Source: CAD feature listing. Evaluate the final solid. Frame: model axes, mm. A direction names the side the tool comes from. Give positions to 0.01 mm unless a question says otherwise; leave off trailing zeros. Loops run counter-clockwise (first coordinate to the right, second up) from the corner with the lowest first, then second, coordinate; pieces in that order, holes last. Notation, with made-up numbers: (46.25, 55.5) - (93.25, 55.5) arc R5 cw to (93.25, 62.5) - close; hole circle Ø7 at (-6, 11). An arc over 180 degrees is marked (long way). Write each question's results on one line, items separated by ' | '. Start each with the question number.
(1) Material intervals for line 1 along Z through (x, y) = (-10.6, 5); line 2 along X through (y, z) = (7, 19.25); line 3 along Y through (x, z) = (10.85, 15), sorted ascending. Write a range as [from, to].
(2) Contact query for flat-ended pins moving along their axis: pin 1 (3.5 mm diameter, centred on x = 0, z = 27, fed in from -Y); pin 2 (3 mm diameter, centred on x = 0.5, z = 26.5, fed in from +Y); pin 3 (1.5 mm diameter, centred on y = 0, z = 27, fed in from +X); pin 4 (1.6 mm diameter, centred on x = -9.5, z = 15, fed in from +Y). Output: stop coordinate, or through.
(3) Pull-direction query (X, two-part tool) for faces 6 (the cylindrical face through (3.4, 0.52, 30.43)), 7 (the cylindrical face through (10.62, 9.289, 6.025)), 8 (the flat face through (0, 1, 22)); classes: pulls with the +X half, pulls with the -X half, needs draft (parallel to the pull), parting line crosses it, or undercut.
(4) Cut plane C-C on x = 1. Return the cut outline in (y, z).
(5) Cut plane D-D on y = 9.25. Return the cut outline in (x, z), then the cut area to 3 significant figures.
(6) Cut plane B-B on y = 5.75. Return the cut outline in (x, z), then the cut area to 3 significant figures.
(7) Reachability of faces 1 (the flat face through (9, 0, 13)), 2 (the flat face through (4, 0, 27)), 3 (the flat face through (-1.396, 1.014, 24.63)), 4 (the flat face through (-1, -1, 23)), 5 (the flat face through (-0.2, 2.4, 23)) from +Z, -Z, +X, -X, +Y, -Y: full face, straight path, thin tool, end or side. Return the list, or none.
(8) Cut plane A-A on z = 14. Return the cut outline in (x, y).
Autodesk Inventor part; units mm, degrees
ref_plane "YZ Plane" through (0, 0, 0) normal (1, 0, 0) x (0, 1, 0)
ref_plane "XZ Plane" through (0, 0, 0) normal (0, 1, 0) x (-1, 0, 0)
ref_plane "XY Plane" through (0, 0, 0) normal (0, 0, 1) x (1, 0, 0)
sketch "Sketch1" plane through (0, 0, 0) normal (0, 1, 0) x (-1, 0, 0)
  line L0 (10.25, 22) -> (-10.25, 22)
  line L1 (-10.25, 22) -> (-10.25, -22)
  line L2 (-10.25, -22) -> (10.25, -22)
  line L3 (10.25, -22) -> (10.25, 22)
  line L4 (10.25, 22) -> (-10.25, -22) construction
  line L5 (-10.25, 22) -> (10.25, -22) construction
  line L6 (-11, 22) -> (11, 22)
  line L7 (11, 22) -> (11, -22)
  line L8 (11, -22) -> (-11, -22)
  line L9 (-11, -22) -> (-11, 22)
  line L10 (-11, 22) -> (11, -22) construction
  line L11 (11, 22) -> (-11, -22) construction
  point P0 (0, 0)
  dimension "d0" = 20.5
  dimension "d1" = 44
  dimension "d2" = 22
extrude "Extrusion1" add sketch "Sketch1" along normal blind 11 contours L6 L7 L8 L3 | L1 L8 L9 L6
sketch "Sketch2" plane through (-11, 0, 22) normal (0, 0, 1) x (1, 0, 0)
  line L0 (0.75, 0) -> (0.75, 11)
  line L1 (0.75, 0) -> (0.75, 11)
  line L2 (0, 11) -> (0.75, 11)
  line L3 (0, 0) -> (0, 11)
  line L4 (0.75, 0) -> (0, 0)
  line L5 (21.25, 11) -> (21.25, 0)
  line L6 (22, 0) -> (21.25, 0)
  line L7 (22, 0) -> (22, 11)
  line L8 (21.25, 11) -> (22, 11)
  line L9 (0, 0) -> (0, 11)
  line L10 (22, 0) -> (22, 11)
  line L11 (0, 0) -> (22, 0)
  line L12 (22, 0) -> (22, 3)
  line L13 (22, 3) -> (0, 3)
  line L14 (0, 3) -> (0, 0)
  point P0 (11, 0)
  dimension "d5" = 3
extrude "Extrusion2" add sketch "Sketch2" along normal blind 1 contours L4 L3 L13 L0 | L0 L13 L5 L11 | L5 L13 L7 L6
mirror "Mirror1" about plane through (0, 0, 0) normal (0, 0, 1) of "Extrusion2"
sketch "Sketch3" plane through (0, 0, 0) normal (0, -1, 0) x (1, 0, 0)
  line L0 (-11, -23) -> (11, -23)
  line L1 (8.25, -23) -> (11, -23)
  line L2 (11, -23) -> (11, 23)
  line L3 (11, 23) -> (8.25, 23)
  line L4 (8.25, 23) -> (8.25, -23)
  line L5 (10.25, 22) -> (10.25, -22)
  line L6 (-10.25, -22) -> (-10.25, 22)
  line L7 (-10.25, 22) -> (10.25, 22)
  line L8 (10.25, 22) -> (10.25, -22)
  line L9 (-10.25, -22) -> (10.25, -22)
  line L10 (-11, 23) -> (-11, -23)
  line L11 (-11, -23) -> (11, -23)
  line L12 (11, -23) -> (11, 23)
  line L13 (-11, 23) -> (11, 23)
  line L14 (-11, -23) -> (-8.25, -23)
  line L15 (-8.25, -23) -> (-8.25, 23)
  line L16 (-8.25, 23) -> (-11, 23)
  line L17 (-11, 23) -> (-11, -23)
  point P0 (0, 0)
  dimension "d9" = 2
  dimension "d10" = 2
extrude "Extrusion3" add sketch "Sketch3" along normal blind 1 contours L10 L13 L15 L7 L6 L9 L0 | L15 L9 L4 L0 | L4 L9 L5 L7 L3 L2 L0 | L9 L6 L7 L15 | L13 L4 L7 L15 | L4 L7 L5 L9
sketch "Sketch4" plane through (11, -1, 23) normal (1, 0, 0) x (0, 0, -1)
  line L0 (1, 4) -> (1, 12)
  line L1 (0, 4) -> (0, 0)
  line L2 (46, 0) -> (0, 0)
  line L3 (46, 0) -> (46, 4)
  line L4 (45, 4) -> (45, 12)
  line L5 (1, 12) -> (45, 12)
  line L6 (45.7791, 4) -> (18.7791, 4)
  line L7 (18.7791, 4) -> (18.7791, 20.689)
  line L8 (18.7791, 20.689) -> (45.7791, 20.689)
  line L9 (45.7791, 20.689) -> (45.7791, 4)
  line L10 (45, 4) -> (46, 4)
  line L11 (1, 4) -> (0, 4)
  point P0 (23, 1)
  dimension "d14" = 27
extrude "Extrusion4" cut sketch "Sketch4" against normal through all contours L7 L8 L9 L6 L4 L5 | L5 L4 L6 L7
sketch "Sketch5" plane through (11, -1, 23) normal (1, 0, 0) x (0, 0, -1)
  point P0 (23, 1)
sketch "Sketch6" plane through (11, -1, 23) normal (1, 0, 0) x (0, 0, -1)
  line L0 (46, 4) -> (18.7791, 4)
  line L1 (18.7791, 4) -> (18.7791, 12)
  line L2 (1, 12) -> (18.7791, 12)
  line L3 (1, 4) -> (1, 12)
  line L4 (0, 4) -> (0, 0)
  line L5 (46, 0) -> (0, 0)
  line L6 (46, 0) -> (46, 4)
  line L7 (18.7791, 8.8707) -> (57.7172, 8.8707)
  line L8 (57.7172, 8.8707) -> (57.7172, -3.4205)
  line L9 (57.7172, -3.4205) -> (18.7791, -3.4205)
  line L10 (18.7791, -3.4205) -> (18.7791, 8.8707)
  line L11 (1, 4) -> (0, 4)
  point P0 (23, 1)
extrude "Extrusion5" cut sketch "Sketch6" against normal through all contours L6 L5 L10 L0 | L0 L1 L7 L8 L9 L10 L5 L6
sketch "Sketch7" plane through (-11, 3, 22) normal (-1, 0, 0) x (0, 0, 1)
  line L0 (1, -4) -> (-17.7791, -4)
  line L1 (1, 0) -> (1, -4)
  point P0 (-22, -3)
  point P1 (-7, 2)
  point P2 (-10, 2)
  dimension "d19" = 6
  dimension "d20" = 6
  dimension "d21" = 8
  dimension "d22" = 3
hole "Hole1" at (-11, 5, 15) at (-11, 5, 12) direction (1, 0, 0) diameter 0.7 end through all
sketch "Sketch8" plane through (0, -1, 0) normal (0, -1, 0) x (1, 0, 0)
  line L0 (-11, 4.2209) -> (-8.25, 4.2209)
  line L1 (-8.25, 22) -> (-8.25, 4.2209)
  line L2 (-8.25, 22) -> (8.25, 22)
  line L3 (8.25, 4.2209) -> (8.25, 22)
  line L4 (8.25, 4.2209) -> (11, 4.2209)
  line L5 (11, 4.2209) -> (11, 23)
  line L6 (11, 23) -> (-11, 23)
  line L7 (-11, 23) -> (-11, 4.2209)
  line L8 (11, 23) -> (-11, 23)
  line L9 (4, 31) -> (-4, 31)
  line L10 (-4, 31) -> (-4, 23)
  line L11 (-4, 23) -> (4, 23)
  line L12 (4, 23) -> (4, 31)
  line L13 (4, 31) -> (-4, 23) construction
  line L14 (-4, 31) -> (4, 23) construction
  point P0 (0, 0)
  point P1 (0, 27)
  dimension "d30" = 8
  dimension "d31" = 0
  dimension "d32" = 8
extrude "Extrusion6" add sketch "Sketch8" against normal blind 3 contours L10 L9 L12 L6
sketch "Sketch9" plane through (-10.25, 3, 22) normal (0, 1, 0) x (1, 0, 0)
  line L0 (20.5, 0) -> (21.25, 0)
  line L1 (20.5, 0) -> (0, 0)
  line L2 (-0.75, 0) -> (0, 0)
  line L3 (-0.75, 0) -> (-0.75, -1)
  line L4 (21.25, -1) -> (-0.75, -1)
  line L5 (21.25, 0) -> (21.25, -1)
  line L6 (7.5011, -6.5896) -> (7.4989, -3.4141)
  line L7 (7.4989, -3.4141) -> (10.2478, -1.8246)
  line L8 (10.2478, -1.8246) -> (12.9989, -3.4104)
  line L9 (12.9989, -3.4104) -> (13.0011, -6.5859)
  line L10 (13.0011, -6.5859) -> (10.2522, -8.1754)
  line L11 (10.2522, -8.1754) -> (7.5011, -6.5896)
  line L12 (6.25, -1) -> (14.25, -1)
  line L13 (6.25, -1) -> (6.25, -9)
  line L14 (6.25, -9) -> (14.25, -9)
  line L15 (14.25, -9) -> (14.25, -1)
  point P0 (10.25, 22)
  point P1 (10.25, -5)
  dimension "d35" = 5.5
  dimension "d38" = 4
extrude "Extrusion7" cut sketch "Sketch9" against normal blind 3 contours L6 L7 L8 L9 L10 L11
sketch "Sketch10" plane through (-10.25, 0, 22) normal (0, 1, 0) x (1, 0, 0)
  line L0 (7.5011, -6.5896) -> (7.4989, -3.4141)
  line L1 (10.2522, -8.1754) -> (7.5011, -6.5896)
  line L2 (13.0011, -6.5859) -> (10.2522, -8.1754)
  line L3 (12.9989, -3.4104) -> (13.0011, -6.5859)
  line L4 (10.2478, -1.8246) -> (12.9989, -3.4104)
  line L5 (7.4989, -3.4141) -> (10.2478, -1.8246)
  point P0 (10.25, 22)
  point P1 (10.2478, -4.9963)
hole "Hole2" at (-0.0022, 0, 26.9963) direction (0, -1, 0) diameter 4 end through all
fillet "Fillet3" radius 2 2 edges at (-4, 0.5, 31) (4, 0.5, 31)
fillet "Fillet4" radius 2 2 edges at (4, 0.5, 23) (-4, 0.5, 23)
fillet "Fillet5" radius 6 4 edges at (-10.625, 11, 22) (10.625, 11, 22) (10.625, 11, 4.2209) (-10.625, 11, 4.2209)
properties part number "protoboard_harness"
Ans:
1) line 1: [4.22, 11.65], [12.35, 14.65], [15.35, 22] | line 2: [-11, -10.25], [10.25, 11] | line 3: [-1, 4.65], [5.35, 11]
2) pin 1: through | pin 2: y = 0 | pin 3: x = 4 | pin 4: y = 11
3) face 6: pulls with the +X half | face 7: needs draft | face 8: undercut
4) outline: (-1, 22) - (3, 22) - (3, 23) - (2, 23) - (2, 24.4) - (0, 24.4) - (0, 25.27) - (-1, 25.27) - close; (-1, 28.73) - (0, 28.73) - (0, 29.6) - (2, 29.6) - (2, 31) - (-1, 31) - close
5) outline: (-11, 5.99) - (-10.25, 5.99) - (-10.25, 20.24) - (-11, 20.24) - close; (10.25, 5.99) - (11, 5.99) - (11, 20.24) - (10.25, 20.24) - close | area: 21.4 mm^2
6) outline: (-11, 4.27) - (-10.25, 4.27) - (-10.25, 21.95) - (-11, 21.95) - close; (10.25, 4.27) - (11, 4.27) - (11, 21.95) - (10.25, 21.95) - close | area: 26.5 mm^2
7) face 1: -Z, +Y | face 2: +Z, +X, +Y, -Y | face 3: +Y | face 4: +Z, -Z, +X, -X, -Y | face 5: +Z, +Y
8) outline: (-11, -1) - (-8.25, -1) - (-8.25, 0) - (-10.25, 0) - (-10.25, 11) - (-11, 11) - close; (8.25, -1) - (11, -1) - (11, 11) - (10.25, 11) - (10.25, 0) - (8.25, 0) - close
